Geometry: see drawing. Coordinates: mm, zero at the bounding-box minimum. A direction names the side the tool comes from. Round coordinates to 2 decimals unless told otherwise and drop trailing zeros. Loops run counter-clockwise (first coordinate to the right, second up) from the corner with the lowest first, then second, coordinate; pieces in that order, holes last.
(1) Section C-C, the plane x = 210. Return the cut outline in (y, z).
(2) Material intervals for probe 1 along Y at (x, z) = (81.5, 21.5); probe 2 along X at (y, z) = (27, 11); probe 3 along X at (y, z) = (46, 9.75), sorted ascending.
(3) Section B-B, the plane y = 29. Return the cut outline in (x, z), plus the area to 3 significant figures.
(4) Set-up query: the marked faces 1 and 2. Return all of +Z, -Z, +X, -X, +Y, -Y with unobstructed straight access to the full face (end or side cutting, diameter ignored); none if empty.
(5) Mould query, pull axis X, two halves, no side actions, for the marked faces 3, 4, 5 and 6. Classes: pulls with the +X half, pulls with the -X half, needs draft (parallel to the pull), parting line crosses it, or undercut.
(6) First-contact query: pin 1 Ø1 at (x, z) = (197.5, 8.5) entering from +Y; pin 2 Ø4 at (y, z) = (30.5, 12) entering from -X. Flat tips, straight axial feed; report the tip coordinate or a pass-through.
(7) Section D-D, the plane x = 114.5. Return the cut outline in (y, z).
(8) Section A-A, the plane z = 12.5. Return the cut outline in (x, y), plus the area to 3 significant figures.
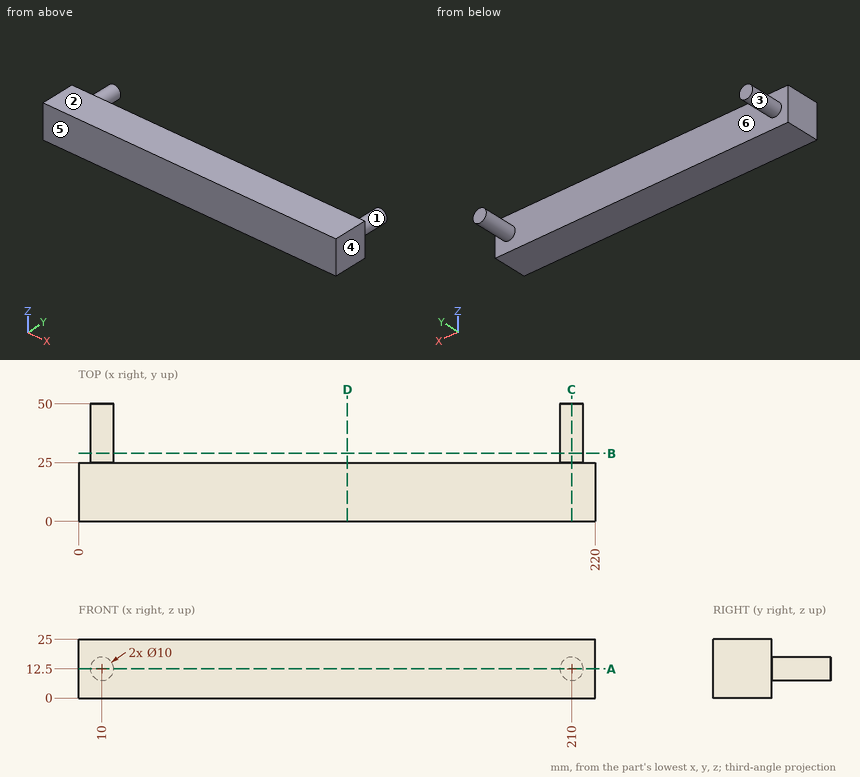
Output values:
1. outline: (0, 0) - (25, 0) - (25, 7.5) - (50, 7.5) - (50, 17.5) - (25, 17.5) - (25, 25) - (0, 25) - close
2. probe 1: y = 0 to 25
2. probe 2: x = 5.23 to 14.77, 205.23 to 214.77
2. probe 3: x = 5.82 to 14.18, 205.82 to 214.18
3. outline: circle Ø10 at (10, 12.5); circle Ø10 at (210, 12.5)
3. area: 157 mm2
4. face 1: +Y
4. face 2: +Z, +X, -X, +Y, -Y
5. face 3: undercut
5. face 4: pulls with the +X half
5. face 5: needs draft
5. face 6: undercut
6. pin 1: stops at y = 25
6. pin 2: stops at x = 5
7. outline: (0, 0) - (25, 0) - (25, 25) - (0, 25) - close
8. outline: (0, 0) - (220, 0) - (220, 25) - (215, 25) - (215, 50) - (205, 50) - (205, 25) - (15, 25) - (15, 50) - (5, 50) - (5, 25) - (0, 25) - close
8. area: 6,000 mm2
